The drawing under review shows one solid part. Ordinate dimensions are in mm from its lowest x, y, z. Round coordinates to 2 decimals unless told otherwise and drop trailing zeros. Loops run counter-clockwise (first coordinate to the right, second up) from the corner with the lowest first, then second, coordinate; pieces in that order, holes last. Notation, with made-up numbers: (-3.5, 42) -> (33.5, 42) arc R27 ccw to (33.5, 78) -> close; hole circle Ø7 at (75, 32). An arc over 180 degrees is marked (long way). Use a Markdown table: item, result. Add a question column.
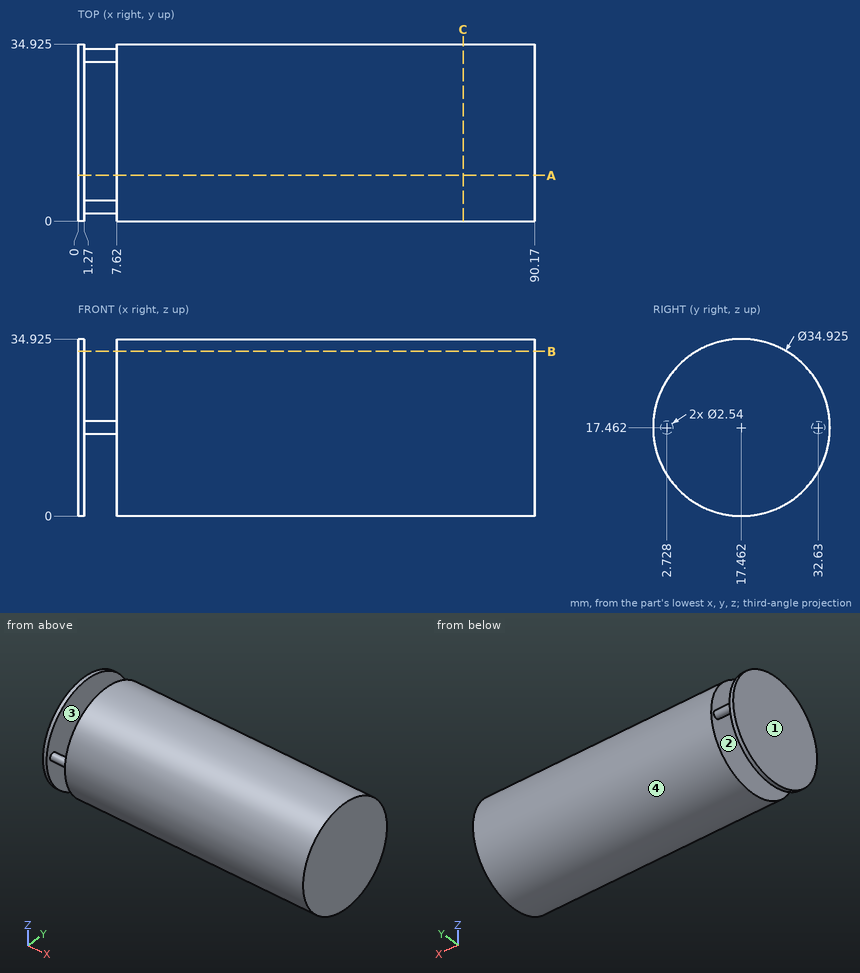
1. To check wall thickness, follow probe 1 along X at (y, z) = (20, 30.5); probe 2 along Z at (x, y) = (33.5, 29) (1 decimal); probe 3 along Y at (x, z) = (38.5, 25.5) (1 decimal). State the ranges of each line that lie inside material, in increasing order. Write a range as from..to.
2. Consider section B-B on z = 32.5. State the section outline as (x, y) points (1 decimal), plus the area to 3 significant figures.
3. Consider section C-C on x = 76. State the section outline as (y, z) points (1 decimal).
4. Consider section A-A on y = 9. State the section outline as (x, z) points.
5. Mouldability with a two-part tool opening along X and no side actions: class the marked faces 1, 2, 3 and 4 as +X half, -X half, draft (parallel to the pull), parting line (faces both ways), or undercut.
6. Insertion check: P1, Ø8, axis at x = 43, z = 5.5, coming from the -Y side; P2, Ø12, axis at x = 12, y = 6.5, coming from the +Z side (1 decimal); P3, Ø1.5, axis at x = 74, y = 25.5, coming from the +Z side. Each pin has a flat end and moves straight along its axis. Give the tip position at first contact, or say it passes through.
Verdict:
| question | item | result |
|---|---|---|
| 1 | probe 1 | x = 0..1.27, 7.62..90.17 |
| 1 | probe 2 | z = 4.4..30.6 |
| 1 | probe 3 | y = 2..33 |
| 2 | outline | (0, 8.6) -> (1.3, 8.6) -> (1.3, 26.3) -> (0, 26.3) -> close; (7.6, 8.6) -> (90.2, 8.6) -> (90.2, 26.3) -> (7.6, 26.3) -> close |
| 2 | area | 1,490 mm² |
| 3 | outline | circle Ø34.9 at (17.5, 17.5) |
| 4 | outline | (0, 2.19) -> (1.27, 2.19) -> (1.27, 32.74) -> (0, 32.74) -> close; (7.62, 2.19) -> (90.17, 2.19) -> (90.17, 32.74) -> (7.62, 32.74) -> close |
| 5 | face 1 | -X half |
| 5 | face 2 | undercut |
| 5 | face 3 | undercut |
| 5 | face 4 | draft |
| 6 | P1 | stops at y = 1.92 |
| 6 | P2 | stops at z = 34.2 |
| 6 | P3 | stops at z = 33.33 |
